from build123d import *

# Parameters (mm, degrees)
SKETCH_1_R                      = 12.55
EXTRUDE_1_DEPTH                 = 8
SKETCH_2_R                      = 3
CUT_EXTRUDE_1_DEPTH             = 7
CUT_EXTRUDE_2_REACH             = 21.468
SKETCH_3_R                      = 1
CUT_EXTRUDE_2_DIRECTION_2_REACH = 21.468
CUT_EXTRUDE_3_DEPTH             = 21
CUT_EXTRUDE_3_DEPTH_BACK        = 19
SKETCH_4_R                      = 1
SKETCH_5_R                      = 13.5
EXTRUDE_2_DEPTH                 = 2.5
SKETCH_6_R                      = 12.5
CUT_EXTRUDE_4_DEPTH             = 2.5
FILLET_1_R                      = 2
SKETCH_7_W                      = 2.5
SKETCH_7_H                      = 6
CUT_EXTRUDE_5_DEPTH             = 21.5


with BuildPart() as part:
    # 草图1 → 凸台-拉伸1 (new body)
    with BuildSketch(Plane(origin=(0, 0, 0), x_dir=(0, 0, -1), z_dir=(1, 0, 0))):
        Circle(SKETCH_1_R)
    extrude(amount=EXTRUDE_1_DEPTH)

    # 草图2 → 切除-拉伸1 (cut)
    with BuildSketch(Plane.ZY):
        Circle(SKETCH_2_R)
    extrude(amount=-CUT_EXTRUDE_1_DEPTH, mode=Mode.SUBTRACT)

    # 草图3 → 切除-拉伸2 (cut, up to next)
    with BuildSketch(Plane(origin=(0, 0, 0), x_dir=(1, 0, 0), z_dir=(0, 1, 0)), mode=Mode.PRIVATE) as cut_extrude_2_sk1:
        with Locations(Location((2, 0, 0), (0, 0, 270))):
            Circle(SKETCH_3_R)
    cut_extrude_2_tool1 = extrude(cut_extrude_2_sk1.sketch, amount=-CUT_EXTRUDE_2_REACH, mode=Mode.PRIVATE) & part.part
    add(cut_extrude_2_tool1.solids().sort_by_distance((2, 0, 0))[0], mode=Mode.SUBTRACT)

    # 草图3 → 切除-拉伸2 direction 2 (cut, up to next)
    with BuildSketch(Plane(origin=(0, 0, 0), x_dir=(1, 0, 0), z_dir=(0, 1, 0)), mode=Mode.PRIVATE) as cut_extrude_2_direction_2_sk1:
        with Locations(Location((2, 0, 0), (0, 0, 270))):
            Circle(SKETCH_3_R)
    cut_extrude_2_direction_2_tool1 = extrude(cut_extrude_2_direction_2_sk1.sketch, amount=CUT_EXTRUDE_2_DIRECTION_2_REACH, mode=Mode.PRIVATE) & part.part
    add(cut_extrude_2_direction_2_tool1.solids().sort_by_distance((2, 0, 0))[0], mode=Mode.SUBTRACT)

    # 草图4 → 切除-拉伸3 (cut, two sides: drawn at the far end of the back side and taken through both)
    with BuildSketch(Plane.XY.offset(-CUT_EXTRUDE_3_DEPTH_BACK)):
        with Locations(Location((5, 0, 0), (0, 0, 180))):
            Circle(SKETCH_4_R)
    extrude(amount=CUT_EXTRUDE_3_DEPTH + CUT_EXTRUDE_3_DEPTH_BACK, mode=Mode.SUBTRACT)

    # 草图5 → 凸台-拉伸2 (add)
    with BuildSketch(Plane(origin=(8, 0, 0), x_dir=(0, 0, -1), z_dir=(1, 0, 0))):
        Circle(SKETCH_5_R)
    extrude(amount=EXTRUDE_2_DEPTH)

    # 草图6 → 切除-拉伸4 (cut)
    with BuildSketch(Plane(origin=(10.5, 0, 0), x_dir=(0, 0, -1), z_dir=(1, 0, 0))):
        Circle(SKETCH_6_R)
    extrude(amount=-CUT_EXTRUDE_4_DEPTH, mode=Mode.SUBTRACT)

    # 圆角1
    # the kernel refuses this fillet: 2 mm, written as the material it adds along each edge
    with BuildSketch(Plane(origin=(8, 0, 0), x_dir=(0, 0, -1), z_dir=(0, -1, 0))) as fillet_1_piece_1:
        with BuildLine():
            CenterArc((14.55, -1.702204453), FILLET_1_R, 121.668243254, 58.331756746)
            Line((12.55, -1.702204453), (12.51, -1.702204453))
            Line((12.51, -1.702204453), (12.51, 0))
            Line((12.51, 0), (12.55, 0.04))
            ThreePointArc((12.55, 0.04), (13.025, 0.04), (13.479, 0.034044089))
            Line((13.479, 0.034044089), (13.5, 0))
        make_face()
    revolve(axis=Axis((8, 0, 0), (1, 0, 0)))

    # 草图7 → 切除-拉伸5 (cut)
    with BuildSketch(Plane.XY):
        with Locations((9.25, 0)):
            Rectangle(SKETCH_7_W, SKETCH_7_H)
    extrude(amount=-CUT_EXTRUDE_5_DEPTH, mode=Mode.SUBTRACT)


solid = part.part
Work out the finished part from the listing and answer in its coordinate system (mm). A direction names the side the tool comes from. Coordinates: 2 decimals unless noted, no trailing zeros. Loops run counter-clockwise (first coordinate to the right, second up) from the corner with the lowest first, then second, coordinate; pieces in that order, holes last. Notation, with made-up numbers: M 20,50.25 L 32,50.25 A15 cw 32,60.25 Z; hole C 56,10.25 d8. An arc over 180 degrees is marked long. Answer in a Markdown table with one row per item. Add a question column.
1. A tool of negligible diameter and unlimited length cuts with its end or side. For faces 1 (the flat face through (9, 3, -13)), 2 (the cylindrical face through (3.1, 3.77, -11.97)), 3 (the flat face through (8, 0, 0)), from which of +Z, -Z, +X, -X, +Y, -Y can it reach the whole face along a straight path? Write none if from no direction.
2. Find section A-A, the plane y = 0. Write down the section's boundary in (x, z).
3. Flat-ended cylindrical pins translate along their axes: P1, Ø2, axis at y = 7, z = -3.5, coming from the +X side; P2, Ø6, axis at x = 4, z = -10.5, coming from the -Y side; P3, Ø5, axis at x = 9.5, z = -4, coming from the +Y side. Find the tip coordinate at first contact, or state that the pin passes through.
4. Find section B-B, the plane z = 0. Write down the section's boundary in (x, y).
5. The mould has two halves that part along X. Classify faces 4 (the cylindrical face through (1, -8, 0)), 5 (the cylindrical face through (9.27, 0.51, 12.49)), 6 (the flat face through (0, -3, -3)), 7 (the cylindrical face through (6, 0, -8)): pulls with the +X half, pulls with the -X half, needs draft (parallel to the pull), parting line crosses it, or undercut.
6. Consider L1, parallel to Y at x = 9, z = 0; L2, parallel to X at y = 4.75, z = 5.5; L3, parallel to Y at x = 2.5, z = -2. Determine where each line is inside the solid, lowest interval first.
7. Find section C-C, the plane x = 2. Write down the section's boundary in (y, z), then the cut area to 3 significant figures.
8. Find section D-D, the plane x = 9.25. Write down the section's boundary in (y, z).
Reported:
| question | item | result |
|---|---|---|
| 1 | face 1 | -Z, +X |
| 1 | face 2 | -X |
| 1 | face 3 | +X |
| 2 | outline | M 0,-12.55 L 4,-12.55 L 4,-3 L 0,-3 Z; M 0,3 L 4,3 L 4,12.55 L 0,12.55 Z; M 6,-12.55 L 6.3,-12.55 A2 cw 8,-13.5 L 8,12.5 L 10.5,12.5 L 10.5,13.5 L 8,13.5 A2 cw 6.3,12.55 L 6,12.55 L 6,3 L 7,3 L 7,-3 L 6,-3 Z |
| 3 | P1 | stops at x = 8 |
| 3 | P2 | stops at y = -10.06 |
| 3 | P3 | stops at y = 13.42 |
| 4 | outline | M 0,-12.55 L 1,-12.55 L 1,-3 L 0,-3 Z; M 0,3 L 1,3 L 1,12.55 L 0,12.55 Z; M 3,-12.55 L 6.3,-12.55 A2 cw 8,-13.5 L 10.5,-13.5 L 10.5,-12.5 L 8,-12.5 L 8,12.5 L 10.5,12.5 L 10.5,13.5 L 8,13.5 A2 cw 6.3,12.55 L 3,12.55 L 3,3 L 7,3 L 7,-3 L 3,-3 Z |
| 5 | face 4 | undercut |
| 5 | face 5 | needs draft |
| 5 | face 6 | pulls with the -X half |
| 5 | face 7 | undercut |
| 6 | L1 | y = -13.5 to -12.5, 12.5 to 13.5 |
| 6 | L2 | x = 0 to 8 |
| 6 | L3 | y = -12.39 to -2.24, 2.24 to 12.39 |
| 7 | outline | M -12.51,-1 A12.55 ccw 12.51,-1 L 2.83,-1 A3 cw -2.83,-1 Z; M -12.51,1 L -2.83,1 A3 cw 2.83,1 L 12.51,1 A12.55 ccw Z |
| 7 | area | 428 mm^2 |
| 8 | outline | M -3,-13.16 L -3,-12.13 A12.5 cw long 3,-12.13 L 3,-13.16 A13.5 ccw long Z |
